```python
from build123d import *

# Parameters (mm, degrees)
BOSS_EXTRUDE1_DEPTH     = 3
ESQUISSE3_R             = 2.35
BOSS_EXTRU_2_DEPTH      = 3
ESQUISSE4_R             = 1
ENL_V_MAT_EXTRU_1_DEPTH = 10
ENL_V_MAT_EXTRU_2_DEPTH = 1.5


with BuildPart() as part:
    # Sketch1 → Boss-Extrude1 (new body)
    with BuildSketch(Plane(origin=(0, 0, 0), x_dir=(1, 0, 0), z_dir=(0, 1, 0))):
        with BuildLine():
            Line((15, 6), (12, 6))
            ThreePointArc((12, 6), (4.759909364, 5.427135296), (-2.3, 3.72279784))
            ThreePointArc((-2.3, 3.72279784), (-5, 0), (-2.3, -3.72279784))
            ThreePointArc((-2.3, -3.72279784), (4.759909364, -5.427135296), (12, -6))
            Line((12, -6), (15, -6))
            Line((15, -6), (15, 6))
        make_face()
    extrude(amount=-BOSS_EXTRUDE1_DEPTH)

    # Esquisse3 → Boss.-Extru.2 (add)
    with BuildSketch(Plane(origin=(0, 0, 0), x_dir=(1, 0, 0), z_dir=(0, 1, 0))):
        with Locations(Location((0, 0, 0), (0, 0, 270))):
            Circle(ESQUISSE3_R)
    extrude(amount=BOSS_EXTRU_2_DEPTH)

    # Esquisse4 → Enlèv. mat.-Extru.1 (cut)
    with BuildSketch(Plane(origin=(0, 0, 0), x_dir=(1, 0, 0), z_dir=(0, 1, 0))):
        with Locations(Location((13.5, -4, 0), (0, 0, 270))):
            Circle(ESQUISSE4_R)
        with Locations(Location((13.5, 4, 0), (0, 0, 270))):
            Circle(ESQUISSE4_R)
    extrude(amount=-ENL_V_MAT_EXTRU_1_DEPTH, mode=Mode.SUBTRACT)

    # Esquisse5 → Enlèv. mat.-Extru.2 (cut)
    with BuildSketch(Plane.XZ.offset(3)):
        with BuildLine():
            Line((13.5, 6.25), (13.5, 10.037760659))
            Line((13.5, 10.037760659), (19.160989733, 10.037760659))
            Line((19.160989733, 10.037760659), (18.711161689, -10.096981605))
            Line((18.711161689, -10.096981605), (13.5, -10.096981605))
            Line((13.5, -10.096981605), (13.5, -6.25))
            ThreePointArc((13.5, -6.25), (11.25, -4), (13.5, -1.75))
            Line((13.5, -1.75), (13.5, 1.75))
            ThreePointArc((13.5, 1.75), (11.25, 4), (13.5, 6.25))
        make_face()
    extrude(amount=-ENL_V_MAT_EXTRU_2_DEPTH, mode=Mode.SUBTRACT)


solid = part.part
```
Verification items for the finished model (mm, model axes). A direction names the side the tool comes from. Round coordinates to 2 decimals unless told otherwise and drop trailing zeros. Order: outer loops, then holes, each group sorted by start corner. A loop starts at its lowest first (then second) coordinate and runs counter-clockwise, first axis right, second up. Notation, with made-up numbers: (74.5, 3.5) - (119.5, 3.5) arc R11 cw to (119.5, 12.5) - close; hole circle Ø8 at (-22, 31). An arc over 180 degrees is marked (long way). Use CSV: the item, a comma, the result in double quotes. Start each with the question number.
1) Thickness scan on L1, parallel to Y at x = 8.75, z = 2.25; L2, parallel to Y at x = 12.5, z = -3; L3, parallel to X at y = 0.15, z = -1. Record the ranges inside material, lowest first.
2) Go/stop test with flat-tipped pins: P1, Ø2, axis at y = -1.5, z = 4.5, coming from the -X side; P2, Ø2.5, axis at x = 13.5, z = -4, coming from the +Y side. Record where each tip stops, or that it passes through.
3) Section check A-A, the plane z = 4.25. Record the cut outline in (x, y), plus the area to 3 significant figures.
4) Access from +Z, -Z, +X, -X, +Y, -Y to the whole of each face (thin tool, end or side, straight path). Record for faces 1 (the cylindrical face through (11.304, -2.26, -3.511)), 2 (the flat face through (13.5, -2, 0)), 3 (the cylindrical face through (0.71, 1.48, 2.24)), 4 (the flat face through (13, -1, 6)).
5) Section check D-D, the plane x = 1.75. Record the cut outline in (y, z), plus the area to 3 significant figures.
6) Mould release check, pull along Z, two halves, no side actions. Record for faces 5 (the cylindrical face through (4.66, -1.48, 5.41)), 6 (the flat face through (14, -1, -6)), 7 (the cylindrical face through (12.524, -0.74, 3.783)): +Z half, -Z half, draft (parallel to the pull), parting line (faces both ways), or undercut.
7) Section check C-C, the plane y = 1.45. Record the cut outline in (x, z), plus the area to 3 significant figures.
8) Section check B-B, the plane z = 0. Record the cut outline in (x, y).
Answers:
1,L1,"y = -3 to 0"
1,L2,"y = -1.5 to 0"
1,L3,"x = -2.13 to 2.13"
2,P1,"stops at x = -2.84"
2,P2,"stops at y = 0"
3,outline,"(-0.57, -3) - (11.26, -3) - (11.26, -1.5) - (12.53, -1.5) - (12.53, 0) - (-0.57, 0) - close; (14.47, -1.5) - (15, -1.5) - (15, 0) - (14.47, 0) - close"
3,area,"38.2 mm²"
4,face 1,"+X, -Y"
4,face 2,"+Z, -Z, +X, -Y"
4,face 3,"+Y"
4,face 4,"+Z, +X, -X, +Y, -Y"
5,outline,"(-3, -4.84) - (0, -4.84) - (0, -1.57) - (3, -1.57) - (3, 1.57) - (0, 1.57) - (0, 4.84) - (-3, 4.84) - close"
5,area,"38.5 mm²"
6,face 5,"+Z half"
6,face 6,"-Z half"
6,face 7,"undercut"
7,outline,"circle Ø4.7 at (0, 0)"
7,area,"17.3 mm²"
8,outline,"(-5, -3) - (13.5, -3) - (13.5, -1.5) - (15, -1.5) - (15, 0) - (2.35, 0) - (2.35, 3) - (-2.35, 3) - (-2.35, 0) - (-5, 0) - close"
